Geometry check sheet. Reference: the model listing, model coordinates, mm. Round coordinates to 2 decimals unless told otherwise and drop trailing zeros. Loops run counter-clockwise (first coordinate to the right, second up) from the corner with the lowest first, then second, coordinate; pieces in that order, holes last. Notation, with made-up numbers: (-29.75, 42) - (22.25, 42) arc R33 ccw to (22.25, 74) - close; hole circle Ø6 at (4.5, 76). An arc over 180 degrees is marked (long way). Answer as CSV lines item,"result". Start each with the question number.
1) Cross-section at B-B on z = 0.7. Record the boundary of the cut face in (x, y) (3 decimals).
2) Thickness scan on line 1 along X through (y, z) = (4.75, 0.8); line 2 along Y through (x, z) = (48, 1.55) (3 decimals); line 3 along X through (y, z) = (2.75, 0.9). Record the ranges inside material, lowest first.
3) Cross-section at C-C on y = 3.25. Record the boundary of the cut face in (x, z), and give its area (3 significant figures).
4) Cross-section at D-D on y = -2.75. Record the boundary of the cut face in (x, z), and give its area (3 significant figures).
5) Cross-section at A-A on x = 48. Record the boundary of the cut face in (y, z) (3 decimals).
6) Depth check by flat-ended pin: P1, Ø7, axis at x = 1.5, y = 1.5, coming from the +Z side; P2, Ø5, axis at x = 73, y = -5, coming from the -Z side; P3, Ø1, axis at y = 0.5, z = 0.5, coming from the +X side; P4, Ø1.5, axis at y = 0, z = 2.5, coming from the -X side. Enter the tip coordinate at first touch or a pass-through.
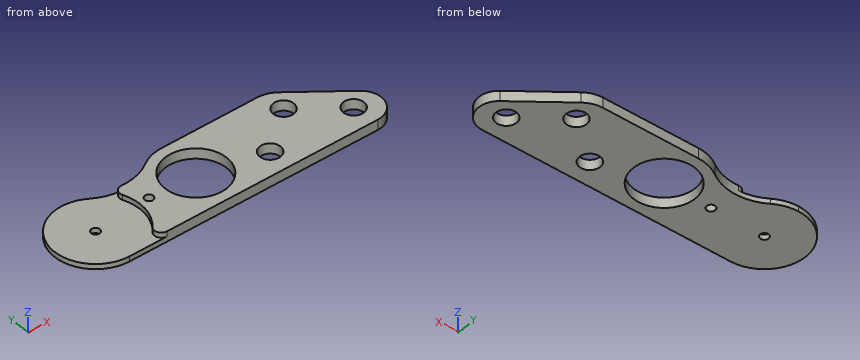
Autodesk Inventor part; units mm, degrees
ref_plane "YZ Plane" through (0, 0, 0) normal (1, 0, 0) x (0, 1, 0)
ref_plane "XZ Plane" through (0, 0, 0) normal (0, 1, 0) x (-1, 0, 0)
ref_plane "XY Plane" through (0, 0, 0) normal (0, 0, 1) x (1, 0, 0)
sketch "スケッチ1" plane through (0, 0, 0) normal (0, 0, 1) x (1, 0, 0)
  line L0 (0, 0) -> (30, 0) construction
  line L1 (0, 12) -> (30, 12)
  line L2 (30, -12) -> (0, -12)
  arc A0 (0, 12) -> (0, -12) centre (0, 0) ccw
  arc A1 (30, -12) -> (30, 12) centre (30, 0) ccw
  circle A2 centre (0, 0) radius 1.25
  circle A3 centre (30, 0) radius 9.025
  arc A4 (6.6667, 9.9778) -> (23.3333, 9.9778) centre (15, 22.4499) ccw
  arc A5 (30, 12) -> (30, -12) centre (30, 0) ccw construction
  arc A6 (0, -12) -> (0, 12) centre (0, 0) ccw construction
  arc A7 (6.6667, 9.9778) -> (0, 12) centre (0, 0) ccw
  arc A8 (30, 12) -> (23.3333, 9.9778) centre (30, 0) ccw
  line L3 (30, 12) -> (92.8308, 12)
  line L4 (92.8308, 12) -> (92.8308, -12)
  line L5 (92.8308, -12) -> (30, -12)
  line L6 (30, -12) -> (30, 12)
  circle A9 centre (16, 0) radius 1.25
  dimension "d0" = 30
  dimension "d1" = 12
  dimension "d2" = 2.5
  dimension "d3" = 18.05
  dimension "d6" = 15
  dimension "d11" = 2.5
  dimension "d12" = 16
extrude "押し出し1" add sketch "スケッチ1" along normal blind 3 contours A7 A4 A8 L6 A3 L2 A0 | L3 L4 L5 A1 | A1 L6 A3
sketch "スケッチ2" plane through (0, 0, 3) normal (0, 0, 1) x (1, 0, 0)
  arc A0 (30, 12) -> (23.3333, 9.9778) centre (30, 0) ccw
  arc A1 (6.6667, 9.9778) -> (23.3333, 9.9778) centre (15, 22.4499) ccw
  arc A2 (6.6667, 9.9778) -> (0, -12) centre (0, 0) ccw
  line L0 (0, -12) -> (92.8308, -12)
  line L1 (92.8308, -12) -> (92.8308, 12)
  line L2 (92.8308, 12) -> (30, 12)
  circle A3 centre (0, 0) radius 1.25
  circle A4 centre (30, 0) radius 9.025
  line L3 (0, -12) -> (92.8308, -12)
  arc A5 (6.6667, 9.9778) -> (23.3333, 9.9778) centre (15, 22.4499) ccw
  arc A6 (0, -12) -> (6.6667, 9.9778) centre (0, 0) ccw
  arc A7 (0, -13) -> (7.8, 10.4) centre (0, 0) ccw
  point P0 (5, -12)
  point P1 (9.9986, 8.3083)
  dimension "d7" = 1
extrude "押し出し2" cut sketch "スケッチ2" against normal blind 1.5 contours A7 L0 A6 A1 | A6 A2
fillet "フィレット1" radius 2 2 edges at (9.9986, 8.3083, 2.25) (5, -12, 2.25)
sketch "スケッチ3" plane through (0, 0, 3) normal (0, 0, 1) x (1, 0, 0)
  arc A0 (30.0122, 16.3221) -> (24.9131, 15.5052) centre (30.0122, 0) ccw
  arc A1 (6.6694, 14.2981) -> (24.9131, 15.5052) centre (15.0061, 26.768) ccw
  arc A2 (6.6694, 14.2981) -> (0, -7.6779) centre (0, 4.3221) ccw
  line L0 (0, -7.6779) -> (30, -7.6779)
  circle A3 centre (0, 0) radius 1.5
  circle A4 centre (16, 0) radius 1.25
  circle A5 centre (48, -5) radius 3.025
  circle A6 centre (73, -5) radius 3.025
  circle A7 centre (60.5, 5) radius 3.025
  line L1 (48, -5) -> (73, -5) construction
  line L2 (61.3547, 12) -> (92.8308, -13.1809)
  line L3 (60.5, 5) -> (73, -5) construction
  line L4 (60.5, 5) -> (60.5, -5) construction
  circle A8 centre (30, 0) radius 9.025
  circle A9 centre (16, 0) radius 1.25
  circle A10 centre (30, 0) radius 9.025
  arc A11 (9.6896, -8.6667) -> (11.1803, -12) centre (11.1803, -10) ccw
  line L5 (11.1803, -12) -> (92.8308, -12)
  line L6 (92.8308, -12) -> (92.8308, 12)
  line L7 (92.8308, 12) -> (30, 12)
  arc A12 (30, 12) -> (23.3333, 9.9778) centre (30, 0) ccw
  arc A13 (14.0846, 7.4779) -> (23.3333, 9.9778) centre (15, 22.4499) ccw
  arc A14 (14.0846, 7.4779) -> (12.1008, 4.7507) centre (13.9625, 5.4816) ccw
  arc A15 (9.6896, -8.6667) -> (12.1008, 4.7507) centre (0, 0) ccw
  line L8 (92.8308, 12) -> (30, 12)
  line L9 (92.8308, -12) -> (92.8308, 12)
  point P0 (60.5, 0)
  point P1 (61.3547, 12)
  point P2 (91.3547, -12)
  point P3 (91.3547, -12)
  dimension "d13" = 6.05
  dimension "d14" = 6.05
  dimension "d15" = 6.05
  dimension "d16" = 25
  dimension "d17" = 10
  dimension "d19" = 6
  dimension "d20" = 18
extrude "押し出し3" cut sketch "スケッチ3" against normal blind 10 contours A5 | A6 | A7 | L7 L6 L5 L2
fillet "フィレット2" radius 8 1 edges at (61.3547, 12, 1.5)
fillet "フィレット3" radius 6 1 edges at (91.3547, -12, 1.5)
properties part number "揺動節"
Answer block:
1,outline,"(0, -12) - (74.25, -12) arc R6 ccw to (77.998, -1.315) - (63.546, 10.247) arc R8 ccw to (58.548, 12) - (30, 12) arc R12.001 ccw to (23.333, 9.978) arc R15 cw to (6.667, 9.978) arc R11.999 ccw to (0, 12) arc R12 ccw to start; hole circle Ø2.5 at (0, 0); hole circle Ø2.5 at (16, 0); hole circle Ø18.05 at (30, 0); hole circle Ø6.05 at (48, -5); hole circle Ø6.05 at (60.5, 5); hole circle Ø6.05 at (73, -5)"
2,line 1,"x = -11.02 to 22.33, 37.67 to 57.49, 63.51 to 70.42"
2,line 2,"y = -12 to -8.025, -1.975 to 12"
2,line 3,"x = -11.68 to 21.4, 38.6 to 58.48, 62.52 to 72.92"
3,outline,"(-11.55, 0) - (21.58, 0) - (21.58, 3) - (12.59, 3) - (12.59, 1.5) - (-11.55, 1.5) - close; (38.42, 0) - (58.03, 0) - (58.03, 3) - (38.42, 3) - close; (62.97, 0) - (72.29, 0) - (72.29, 3) - (62.97, 3) - close"
3,area,"150 mm^2"
4,outline,"(-11.68, 0) - (21.4, 0) - (21.4, 3) - (12.71, 3) - (12.71, 1.5) - (-11.68, 1.5) - close; (38.6, 0) - (45.98, 0) - (45.98, 3) - (38.6, 3) - close; (50.02, 0) - (70.98, 0) - (70.98, 3) - (50.02, 3) - close; (75.02, 0) - (79.29, 0) - (79.29, 3) - (75.02, 3) - close"
4,area,"161 mm^2"
5,outline,"(-12, 0) - (-8.025, 0) - (-8.025, 3) - (-12, 3) - close; (-1.975, 0) - (12, 0) - (12, 3) - (-1.975, 3) - close"
6,P1,"stops at z = 1.5"
6,P2,"passes through"
6,P3,"stops at x = 76.35"
6,P4,"stops at x = 12.98"
